Verification items for the finished model (mm, model axes). Face numbers are marked on the shaded views. A direction names the side the tool comes from. Coordinates: 2 decimals unless noted, no trailing zeros. Order: outer loops, then holes, each group sorted by start corner. A loop starts at its lowest first (then second) coordinate and runs counter-clockwise, first axis right, second up. Notation, with made-up numbers: M 13,52.5 L 18,52.5 A25 ccw 18,76.5 Z; hole C 58.25,54 d1. An arc over 180 degrees is marked long. Answer as a JSON object with one key per item and string values. Group by question number.
(1) Cross-section at A-A (z = -22). Enter the section's corners in (x, y), plus the area to 3 significant figures.
(2) Cross-section at C-C (x = 18). Enter the section's corners in (y, z).
(3) Cross-section at D-D (x = -68). Enter the section's corners in (y, z).
(4) Access from +Z, -Z, +X, -X, +Y, -Y to the whole of each face (thin tool, end or side, straight path). Record for the marked faces 4 and 5.
(5) Cross-section at B-B (y = 39). Enter the section's corners in (x, z).
(6) Mould release check, pull along Z, two halves, no side actions. Record for the marked faces 1, 2 and 3: released by +Z, released by -Z, zero draft, split by the parting line, or undercut.
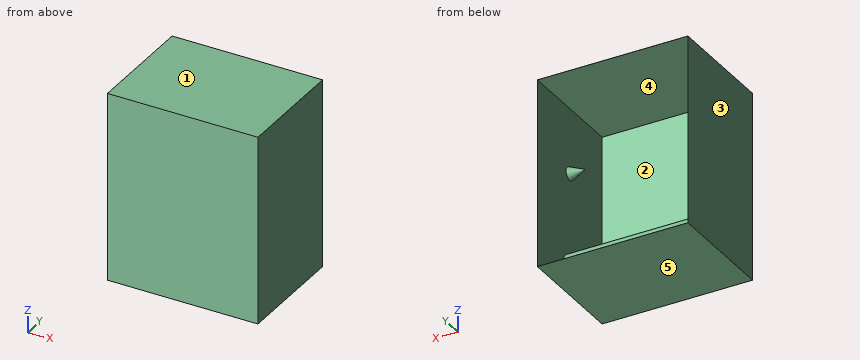
from build123d import *

# Parameters (mm, degrees)
SKETCH1_W               = 160
SKETCH1_H               = 200
BOSS_EXTRUDE1_DEPTH     = 120
SHELL1_T                = 0.1
BOSS_EXTRUDE2_START     = -160
BOSS_EXTRUDE2_OUTLINE_R = 12.5
BOSS_EXTRUDE2_DEPTH     = 159.9
FILLET3_R               = 0.1


# Read off the part's stored shape, not the designer's step: Boss-Extrude2
with BuildPart() as part:
    # Sketch1 → Boss-Extrude1 (new body)
    with BuildSketch(Plane(origin=(0, 0, 0), x_dir=(1, 0, 0), z_dir=(0, 1, 0))):
        with Locations((0, 3.38028169)):
            Rectangle(SKETCH1_W, SKETCH1_H)
    extrude(amount=BOSS_EXTRUDE1_DEPTH)

    # Shell1
    shell1_openings = [part.faces().sort_by_distance(p)[0] for p in [
        (0, 120, -3.38028169),
    ]]
    offset(amount=SHELL1_T, openings=shell1_openings, kind=Kind.INTERSECTION)

    # Boss-Extrude2 outline → Boss-Extrude2 (add)
    with BuildSketch(Plane(origin=(80.1, 0, 0), x_dir=(0, 0, -1), z_dir=(1, 0, 0)).offset(BOSS_EXTRUDE2_START)):
        with Locations((73.48028169, 59.62639051)):
            Circle(BOSS_EXTRUDE2_OUTLINE_R)
    extrude(amount=BOSS_EXTRUDE2_DEPTH)

    # Fillet3
    fillet3_edges = [part.edges().sort_by_distance(p)[0] for p in [
        (80.1, 59.95, -103.48028169),
        (80.1, 59.95, 96.71971831),
        (-80.1, 59.95, 96.71971831),
        (-80.1, 59.95, -103.48028169),
    ]]
    fillet(fillet3_edges, radius=FILLET3_R)

    # Boss-Extrude3 cone 1 section (through the dimple's axis) → Boss-Extrude3 (revolve)
    with BuildSketch(Plane(origin=(-80.1, 60, 26.61971831), x_dir=(0, 0, 1), z_dir=(0, 1, 0))):
        Polygon((0, 0), (7, 0), (0, 16.490966561), align=None)
    revolve(axis=Axis((-80.1, 60, 26.61971831), (1, 0, 0)))

    # Boss-Extrude4 cone 1 section (through the dimple's axis) → Boss-Extrude4 (revolve)
    with BuildSketch(Plane(origin=(80, 60, 26.61971831), x_dir=(0, 0, -1), z_dir=(0, 1, 0))):
        Polygon((0, 0), (7, 0), (0, 16.490966561), align=None)
    revolve(axis=Axis((80, 60, 26.61971831), (-1, 0, 0)))


solid = part.part
Taken from the geometry:
{
 "1": {"outline": "M -80.1,-0.1 L 80.1,-0.1 L 80.1,120 L 80,120 L 80,0 L -80,0 L -80,120 L -80.1,120 Z", "area": "40.0 mm²"},
 "2": {"outline": "M -0.1,-103.48 L 120,-103.48 L 120,-103.38 L 0,-103.38 L 0,96.62 L 120,96.62 L 120,96.72 L -0.1,96.72 Z; C 59.63,-73.48 d25"},
 "3": {"outline": "M -0.1,-103.48 L 120,-103.48 L 120,-103.38 L 0,-103.38 L 0,96.62 L 120,96.62 L 120,96.72 L -0.1,96.72 Z; C 59.63,-73.48 d25; C 60,26.62 d3.73"},
 "4": {"face 4": "+Y", "face 5": "-Z, +X, -X, +Y, -Y"},
 "5": {"outline": "M -80.1,-103.38 A0.1 ccw -80,-103.48 L 80,-103.48 A0.1 ccw 80.1,-103.38 L 80.1,96.62 A0.1 ccw 80,96.72 L -80,96.72 A0.1 ccw -80.1,96.62 Z; hole M -80,-103.38 L 80,-103.38 L 80,96.62 L -80,96.62 Z"},
 "6": {"face 1": "released by +Z", "face 2": "undercut", "face 3": "zero draft"}
}
